```python
from build123d import *

# Parameters (mm, degrees)
F1_DEPTH = 1
F2_R     = 0.6
F3_DEPTH = 25
F5_DEPTH = 0.4
F7_DEPTH = 0.6


with BuildPart() as f1:
    # F0 (on Top) → F1 (new body)
    with BuildSketch(Plane.XY):
        with BuildLine():
            Line((0, 11.298485), (-1.644133, 4.721951))
            ThreePointArc((-1.644133, 4.721951), (-2.5, 4.330127), (-3.267263, 3.784837))
            Line((-3.267263, 3.784837), (-8.035331, 4.6392))
            Line((-8.035331, 4.6392), (-4.978388, 0.923433))
            Line((-4.978388, 0.923433), (-4.92561, 0.859281))
            ThreePointArc((-4.92561, 0.859281), (-5, 0), (-4.92561, -0.859281))
            Line((-4.92561, -0.859281), (-4.978388, -0.923433))
            Line((-4.978388, -0.923433), (-8.035331, -4.6392))
            Line((-8.035331, -4.6392), (-3.288911, -3.849694))
            Line((-3.288911, -3.849694), (-3.206964, -3.836063))
            ThreePointArc((-3.206964, -3.836063), (-2.5, -4.330127), (-1.718646, -4.695344))
            Line((-1.718646, -4.695344), (-1.689478, -4.773127))
            Line((-1.689478, -4.773127), (0, -9.278401))
            Line((0, -9.278401), (1.689478, -4.773127))
            Line((1.689478, -4.773127), (1.718646, -4.695344))
            ThreePointArc((1.718646, -4.695344), (2.5, -4.330127), (3.206964, -3.836063))
            Line((3.206964, -3.836063), (3.288911, -3.849694))
            Line((3.288911, -3.849694), (8.035331, -4.6392))
            Line((8.035331, -4.6392), (4.978388, -0.923433))
            Line((4.978388, -0.923433), (4.92561, -0.859281))
            ThreePointArc((4.92561, -0.859281), (5, 0), (4.92561, 0.859281))
            Line((4.92561, 0.859281), (4.978388, 0.923433))
            Line((4.978388, 0.923433), (8.035331, 4.6392))
            Line((8.035331, 4.6392), (3.288911, 3.849694))
            Line((3.288911, 3.849694), (3.206964, 3.836063))
            ThreePointArc((3.206964, 3.836063), (2.465661, 4.349772), (1.644133, 4.721951))
            Line((1.644133, 4.721951), (0, 11.298485))
        make_face()
        Polygon((-4.705127, -1.850481), (-3.955127, -3.149519), (-6.928203, -4), align=None, mode=Mode.SUBTRACT)
        Polygon((-0.75, -5), (0.75, -5), (0, -8), align=None, mode=Mode.SUBTRACT)
        Polygon((3.955127, -3.149519), (4.705127, -1.850481), (6.928203, -4), align=None, mode=Mode.SUBTRACT)
        Polygon((-3.955127, 3.149519), (-4.705127, 1.850481), (-6.928203, 4), align=None, mode=Mode.SUBTRACT)
        Polygon((4.705127, 1.850481), (3.955127, 3.149519), (6.928203, 4), align=None, mode=Mode.SUBTRACT)
        Polygon((-0.75, 5), (0, 8), (0.75, 5), align=None, mode=Mode.SUBTRACT)
        with BuildLine():
            ThreePointArc((-3.267263, 3.784837), (-2.5, 4.330127), (-1.644133, 4.721951))
            Line((-1.644133, 4.721951), (-4.75, 8.227241))
            Line((-4.75, 8.227241), (-3.267263, 3.784837))
        make_face()
        with BuildLine():
            Line((4.75, 8.227241), (1.644133, 4.721951))
            ThreePointArc((1.644133, 4.721951), (2.465661, 4.349772), (3.206964, 3.836063))
            Line((3.206964, 3.836063), (3.288911, 3.849694))
            Line((3.288911, 3.849694), (4.75, 8.227241))
        make_face()
        with BuildLine():
            Line((-4.92561, 0.859281), (-4.978388, 0.923433))
            Line((-4.978388, 0.923433), (-9.5, 0))
            Line((-9.5, 0), (-4.978388, -0.923433))
            Line((-4.978388, -0.923433), (-4.92561, -0.859281))
            ThreePointArc((-4.92561, -0.859281), (-5, 0), (-4.92561, 0.859281))
        make_face()
        with BuildLine():
            Line((9.5, 0), (4.978388, 0.923433))
            Line((4.978388, 0.923433), (4.92561, 0.859281))
            ThreePointArc((4.92561, 0.859281), (5, 0), (4.92561, -0.859281))
            Line((4.92561, -0.859281), (4.978388, -0.923433))
            Line((4.978388, -0.923433), (9.5, 0))
        make_face()
        with BuildLine():
            Line((-3.206964, -3.836063), (-3.288911, -3.849694))
            Line((-3.288911, -3.849694), (-4.75, -8.227241))
            Line((-4.75, -8.227241), (-1.689478, -4.773127))
            Line((-1.689478, -4.773127), (-1.718646, -4.695344))
            ThreePointArc((-1.718646, -4.695344), (-2.5, -4.330127), (-3.206964, -3.836063))
        make_face()
        with BuildLine():
            Line((4.75, -8.227241), (3.288911, -3.849694))
            Line((3.288911, -3.849694), (3.206964, -3.836063))
            ThreePointArc((3.206964, -3.836063), (2.5, -4.330127), (1.718646, -4.695344))
            Line((1.718646, -4.695344), (1.689478, -4.773127))
            Line((1.689478, -4.773127), (4.75, -8.227241))
        make_face()
    extrude(amount=F1_DEPTH)

    # F2 (on face) → F3 (cut)
    with BuildSketch(Plane.XY.offset(1)):
        Polygon((0.75, 5), (-0.75, 5), (0, 3.4), align=None)
        Polygon((2.365272, 4.096771), (0.69282, 3), (0.69282, 1.2), (2.251666, 2.1), align=None)
        Polygon((-2.944486, 1.7), (-3.955127, 3.149519), (-4.705127, 1.850481), align=None)
        Polygon((-0.69282, 3), (-2.365272, 4.096771), (-2.251666, 2.1), (-0.69282, 1.2), align=None)
        Polygon((-2.944486, -1.7), (-4.705127, -1.850481), (-3.955127, -3.149519), align=None)
        Polygon((-2.944486, 0.9), (-4.730543, 0), (-2.944486, -0.9), (-1.385641, 0), align=None)
        Polygon((0, -3.4), (-0.75, -5), (0.75, -5), align=None)
        Polygon((-2.251666, -2.1), (-2.365272, -4.096771), (-0.69282, -3), (-0.69282, -1.2), align=None)
        Polygon((2.944486, -1.7), (3.955127, -3.149519), (4.705127, -1.850481), align=None)
        Polygon((0.69282, -3), (2.365272, -4.096771), (2.251666, -2.1), (0.69282, -1.2), align=None)
        Polygon((2.944486, 1.7), (4.705127, 1.850481), (3.955127, 3.149519), align=None)
        Polygon((2.944486, -0.9), (4.730543, 0), (2.944486, 0.9), (1.385641, 0), align=None)
        Circle(F2_R)
    extrude(amount=-F3_DEPTH, mode=Mode.SUBTRACT)

    # F4 (on face) → F5 (cut)
    with BuildSketch(Plane.XY.offset(1)):
        Polygon((0, 2.545658), (-0.69282, 3), (-0.69282, 1.2), (-2.251666, 2.1), (-2.204604, 1.272829), (-2.944486, 0.9), (-1.385641, 0), (-2.944486, -0.9), (-2.204604, -1.272829), (-2.251666, -2.1), (-0.69282, -1.2), (-0.69282, -3), (0, -2.545658), (0.69282, -3), (0.69282, -1.2), (2.251666, -2.1), (2.204604, -1.272829), (2.944486, -0.9), (1.385641, 0), (2.944486, 0.9), (2.204604, 1.272829), (2.251666, 2.1), (0.69282, 1.2), (0.69282, 3), align=None)
    extrude(amount=-F5_DEPTH, mode=Mode.SUBTRACT)

    # F6 (on Top) → F7 (join)
    with BuildSketch(Plane.XY):
        Polygon((-2.311537, 7.120197), (-5.010503, 5.561948), (-3.211192, 5.561948), align=None)
        Polygon((-7.32204, 1.558248), (-7.32204, -1.558248), (-6.422384, 0), align=None)
        Polygon((-5.010503, -5.561948), (-2.311537, -7.120197), (-3.211192, -5.561948), align=None)
        Polygon((2.311537, -7.120197), (5.010503, -5.561948), (3.211192, -5.561948), align=None)
        Polygon((7.32204, -1.558248), (7.32204, 1.558248), (6.422384, 0), align=None)
        Polygon((5.010503, 5.561948), (2.311537, 7.120197), (3.211192, 5.561948), align=None)
    extrude(amount=F7_DEPTH)


solid = f1.part
```
Could you check a few things on this model? Use its own coordinates, in mm. A direction names the side the tool comes from. Coordinates: 2 decimals unless noted, no trailing zeros. Write each loop counter-clockwise with the first axis right and the second up, starting at its lowest first coordinate (ties: lowest second). Pieces come first, ordered by that corner, then holes. Notation, with made-up numbers: (0, 29) -> (13, 29) arc R16 ccw to (13, 36) -> close; hole circle Ø4 at (15, -8.75). An arc over 180 degrees is marked (long way). One line per question, with ' | ' between items. Start each with the question number.
1. For faces 1 (the face through (-0.86, -6.99, 0.49)), 2 (the face through (1.461, 1.644, 0.304)), 3 (the face through (0.834, 7.964, 0.493)), 4 (the face through (2.8, -6.6, 0.6)), which set-ups out of +Z, -Z, +X, -X, +Y, -Y let a thin tool reach every point of the face, with its end or its side?
2. If we section it at C-C (x = -5.75): Please give me the cut outline in (y, z).
3. If we section it at A-A (x = 5.5): Please give me the cut outline in (y, z), and give its area (3 significant figures).
4. Please list where these lines run through material, in increasing order: line 1 along X through (y, z) = (7.25, 0.65); line 2 along X through (y, z) = (1, 0.55); line 3 along Y through (x, z) = (-7.5, 0.6).
5. If we section it at B-B (z = 0.85): Count the separate pieces of the cut face and the enclosed holes in it, and give its area (3 significant figures).
6. Thinking about a two-plate mould opening in X: for faces 5 (the face through (1, 0, 0)), 6 (the face through (-5.8, 2.91, 0.49)), which applies, pulls with the +X half, pulls with the -X half, needs draft (parallel to the pull), parting line crosses it, or undercut?
7. Will these pins go through, and if not, where does the flat tip stop? P1, Ø0.5, axis at y = 1, z = 0, coming from the +X side; P2, Ø0.5, axis at x = 7, y = -1, coming from the +Z side; P3, Ø0.5, axis at y = -2.5, z = 0.5, coming from the +X side.
Return value:
1) face 1: +Z, -Z, -Y | face 2: +Z, -Z | face 3: +Z, -Z, +Y | face 4: +Z, -Y
2) outline: (-4.26, 0) -> (-3.66, 0) -> (-3.66, 1) -> (-4.26, 1) -> close; (-2.86, 0) -> (-1.86, 0) -> (-1.86, 1) -> (-2.86, 1) -> close; (-0.77, 0) -> (0.77, 0) -> (0.77, 1) -> (-0.77, 1) -> close; (1.86, 0) -> (2.86, 0) -> (2.86, 1) -> (1.86, 1) -> close; (3.66, 0) -> (4.23, 0) -> (4.23, 1) -> (3.66, 1) -> close
3) outline: (-4.22, 0) -> (-3.59, 0) -> (-3.59, 1) -> (-4.22, 1) -> close; (-2.62, 0) -> (-1.56, 0) -> (-1.56, 1) -> (-2.62, 1) -> close; (-0.82, 0) -> (0.82, 0) -> (0.82, 1) -> (-0.82, 1) -> close; (1.56, 0) -> (2.62, 0) -> (2.62, 1) -> (1.56, 1) -> close; (3.59, 0) -> (4.22, 0) -> (4.22, 1) -> (3.59, 1) -> close | area: 5.01 mm²
4) line 1: x = -4.42 to -3.88, -1.01 to -0.19, 0.19 to 1.01, 3.88 to 4.42 | line 2: x = -7.32 to -7, -5.04 to 5.04, 7 to 7.32 | line 3: y = -4.55 to -3.99, -0.41 to 0.41, 3.99 to 4.54
5) separate pieces: 1 | enclosed holes: 7 | area: 92.7 mm²
6) face 5: needs draft | face 6: undercut
7) P1: stops at x = 7.32 | P2: stops at z = 0.6 | P3: stops at x = 6.48
